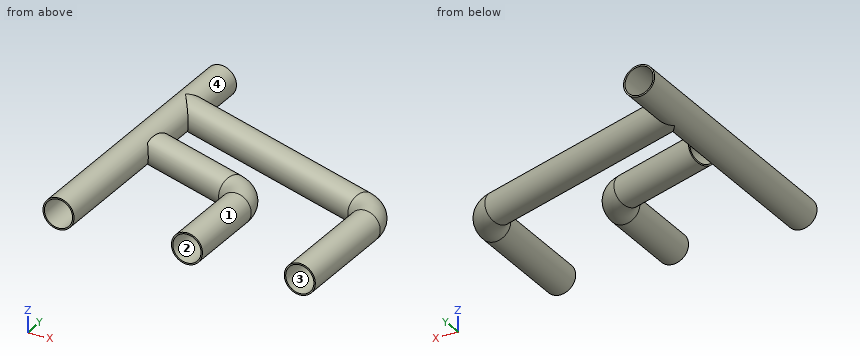
from build123d import *

# Parameters (mm, degrees)
SKETCH1_R                = 6.985
SKETCH1_R_2              = 6.35
BOSS_EXTRUDE1_DEPTH      = 127
SKETCH3_R                = 6.985
SKETCH3_R_2              = 6.35
BOSS_EXTRUDE3_REACH      = 171.672
BOSS_EXTRUDE3_END_RADIUS = 6.985
SKETCH6_R                = 6.985
SKETCH9_R                = 6.985
SKETCH9_R_2              = 6.35


with BuildPart() as part:
    # Sketch1 → Boss-Extrude1 (new body)
    with BuildSketch(Plane(origin=(0, 0, 0), x_dir=(1, 0, 0), z_dir=(0, 1, 0))):
        with Locations(Location((0, 0, 0), (0, 0, 270))):
            Circle(SKETCH1_R)
        with Locations(Location((0, 0, 0), (0, 0, 270))):
            Circle(SKETCH1_R_2, mode=Mode.SUBTRACT)
    extrude(amount=BOSS_EXTRUDE1_DEPTH)



with BuildPart() as body_2:
    # Sweep10: sweep along a path in Sketch2
    with BuildLine(Plane.XY) as sweep10_path:
        Line((108.585, 0), (108.585, 50.8))
        ThreePointArc((108.585, 50.8), (106.288230962, 58.084420742), (100.22865582, 62.734096284))
    # Sketch3 → Sweep10 (sweep)
    with BuildSketch(Plane(origin=(108.585, 0, 0), x_dir=(-1, 0, 0), z_dir=(0, -1, 0))):
        Circle(SKETCH3_R)
        Circle(SKETCH3_R_2, mode=Mode.SUBTRACT)
    sweep(path=sweep10_path.line)


with BuildPart() as part_1:
    add(part.part)

    add(body_2.part)  # Boss-Extrude3 merges body 2
    # Boss-Extrude3: up to this cylinder (the profile starts outside it)
    boss_extrude3_end = Plane(origin=(0, 62.734096, 0), z_dir=(0, -1, 0)) * Cylinder(BOSS_EXTRUDE3_END_RADIUS, 358.314, mode=Mode.PRIVATE)
    # Sketch6 → Boss-Extrude3 (add, up to the surface)
    with BuildSketch(Plane(origin=(68.341780428, -24.874373833, 0), x_dir=(0, 0, 1), z_dir=(-0.9396926207859093, 0.3420201433256665, 0)), mode=Mode.PRIVATE) as boss_extrude3_sk1:
        with Locations(Location((0, 93.230986579, 0), (0, 0, 90))):
            Circle(SKETCH6_R)
    boss_extrude3_tool1 = extrude(boss_extrude3_sk1.sketch, amount=BOSS_EXTRUDE3_REACH, mode=Mode.PRIVATE) - boss_extrude3_end
    add(boss_extrude3_tool1.solids().sort_by_distance((100.228656, 62.734096, 0))[0])

    # Sweep14: sweep along a path in Sketch8
    with BuildLine(Plane.XY) as sweep14_path:
        Line((6.985, 65.482323636), (49.42865582, 50.034096284))
        ThreePointArc((49.42865582, 50.034096284), (55.488230962, 45.384420742), (57.785, 38.1))
        Line((57.785, 38.1), (57.785, 0))
    # Sketch9 → Sweep14 (sweep)
    with BuildSketch(Plane(origin=(57.785, 0, 0), x_dir=(-1, 0, 0), z_dir=(0, -1, 0))):
        Circle(SKETCH9_R)
        Circle(SKETCH9_R_2, mode=Mode.SUBTRACT)
    sweep(path=sweep14_path.line)


solid = part_1.part
Geometry: final body of the model. Coordinates: model frame, mm. Face numbers are marked on the shaded views. A direction names the side the tool comes from. Give positions to 0.01 mm unless a question says otherwise; leave off trailing zeros. Write each loop counter-clockwise with the first axis right and the second up, starting at its lowest first coordinate (ties: lowest second). Pieces come first, ordered by that corner, then holes. Notation, with made-up numbers: (18, 51) -> (24, 51) arc R15 ccw to (24, 66) -> close; hole circle Ø6 at (-38, 25.5). An arc over 180 degrees is marked (long way). Answer in a Markdown table with one row per item.
(1) Pin query (flat end, axial travel): pin 1 (1 mm diameter, centred on y = 36, z = -4.5, fed in from +X); pin 2 (6 mm diameter, centred on x = 43.5, y = 77, fed in from +Z); pin 3 (8 mm diameter, centred on x = 51.5, z = -4, fed in from +Y). Return the tip coordinate at first contact, or that it passes through.
Answers below:
| item | result |
|---|---|
| pin 1 | x = 114.31 |
| pin 2 | z = 6.31 |
| pin 3 | y = 88.87 |
(2) Ray query, line 1 along X through (y, z) = (24, 3.5); line 2 along Z through (x, y) = (54, 48); line 3 along Y through (x, z) = (49, 0.25). Return the intervals inside material, ascending. Write a range as [from, to].
Answers below:
| item | result |
|---|---|
| line 1 | [-6.04, -5.3], [5.3, 6.04], [51.74, 52.49], [63.08, 63.83], [102.54, 103.29], [113.88, 114.63] |
| line 2 | [-6.96, -6.32], [6.32, 6.96] |
| line 3 | [42.27, 43.11], [56.94, 57.62], [73.95, 88.81] |
(3) Draft query along Z for the marked faces 1 and 2. Return one class per face: +Z half, -Z half, draft (parallel to the pull), parting line (faces both ways), or undercut.
Answers below:
| item | result |
|---|---|
| face 1 | parting line |
| face 2 | undercut |
(4) Section query A-A on y = 29. Return loops of the section in (x, z) (3 decimals).
Answers below:
| item | result |
|---|---|
| outline | circle Ø13.97 at (0, 0); circle Ø13.97 at (57.785, 0); circle Ø13.97 at (108.585, 0); hole circle Ø12.7 at (0, 0); hole circle Ø12.7 at (57.785, 0); hole circle Ø12.7 at (108.585, 0) |
(5) Section query B-B on z = -1.75. State how many separate pieces and enclosed holes the cut face has, then the cut area to 3 significant figures.
Answers below:
| item | result |
|---|---|
| separate pieces | 3 |
| enclosed holes | 0 |
| area | 1,730 mm^2 |
(6) Set-up query: the marked faces 3 and 4. Return all of +Z, -Z, +X, -X, +Y, -Y with unobstructed straight access to the full face (end or side cutting, diameter ignored); none if empty.
Answers below:
| item | result |
|---|---|
| face 3 | -Y |
| face 4 | none |
